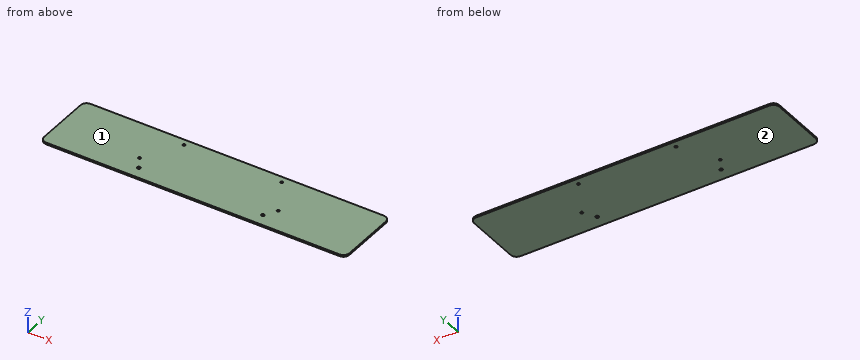
```python
from build123d import *

# Parameters (mm, degrees)
SKETCH1_W           = 500
SKETCH1_H           = 110
BOSS_EXTRUDE1_DEPTH = 3
SKETCH2_R           = 2.65
SKETCH2_R_2         = 2.125
CUT_EXTRUDE1_DEPTH  = 10
SKETCH3_R           = 2.125
CUT_EXTRUDE2_DEPTH  = 10
FILLET1_R           = 10


with BuildPart() as part:
    # Sketch1 → Boss-Extrude1 (new body)
    with BuildSketch(Plane.XY):
        with Locations((250, 55)):
            Rectangle(SKETCH1_W, SKETCH1_H)
    extrude(amount=BOSS_EXTRUDE1_DEPTH)

    # Sketch2 → Cut-Extrude1 (cut)
    with BuildSketch(Plane.XY.offset(3)):
        with Locations((148.5, 20)):
            Circle(SKETCH2_R)
        with Locations((136.5, 40)):
            Circle(SKETCH2_R_2)
        with Locations(Location((363.5, 40, 0), (0, 0, 180))):
            Circle(SKETCH2_R_2)
        with Locations(Location((351.5, 20, 0), (0, 0, 180))):
            Circle(SKETCH2_R)
    extrude(amount=-CUT_EXTRUDE1_DEPTH, mode=Mode.SUBTRACT)

    # Sketch3 → Cut-Extrude2 (cut)
    with BuildSketch(Plane.XY.offset(3)):
        with Locations((170, 99.2)):
            Circle(SKETCH3_R)
        with Locations(Location((330, 99.2, 0), (0, 0, 180))):
            Circle(SKETCH3_R)
    extrude(amount=-CUT_EXTRUDE2_DEPTH, mode=Mode.SUBTRACT)

    # Fillet1
    fillet1_edges = [part.edges().sort_by_distance(p)[0] for p in [
        (0, 110, 1.5),
        (500, 110, 1.5),
        (500, 0, 1.5),
        (0, 0, 1.5),
    ]]
    fillet(fillet1_edges, radius=FILLET1_R)


solid = part.part
```
Read the model definition and answer for the solid it produces. Units are mm, in the model's axes. Face numbers are marked on the shaded views. Round coordinates to 2 decimals unless told otherwise and drop trailing zeros. Use CSV: the item, a comma, the result in double quotes.
Q1. Straight lines are drawn through the part: line 1 along Y through (x, z) = (136.5, 2.05) (3 decimals); line 2 along Y through (x, z) = (351.5, 0.9); line 3 along X through (y, z) = (7.5, 2.65). For each, find the intervals that lie inside material, in ascending order.
Values:
line 1,"y = 0 to 37.875, 42.125 to 110"
line 2,"y = 0 to 17.35, 22.65 to 110"
line 3,"x = 0.32 to 499.68"
Q2. This flat-tipped pin is pushed along its axis until it touches: pin 1 Ø2.5 at (x, y) = (170, 99.2) entering from -Z. Where does it stop, or does it pass through?
Values:
pin 1,"passes through"
Q3. Determine the mould class of the marked faces 1 and 2 for opening direction Z: +Z half, -Z half, draft (parallel to the pull), parting line (faces both ways), or undercut.
Values:
face 1,"+Z half"
face 2,"-Z half"
